Autodesk Inventor part; units mm, degrees
ref_plane "YZ Plane" through (0, 0, 0) normal (1, 0, 0) x (0, 1, 0)
ref_plane "XZ Plane" through (0, 0, 0) normal (0, 1, 0) x (-1, 0, 0)
ref_plane "XY Plane" through (0, 0, 0) normal (0, 0, 1) x (1, 0, 0)
sketch "Sketch1" plane through (0, 0, 0) normal (1, 0, 0) x (0, 1, 0)
  line L0 (2.5746, 9.4872) -> (-17.4254, 9.4872)
  line L1 (-17.4254, 9.4872) -> (-17.4254, -4.5128)
  line L2 (-17.4254, -4.5128) -> (2.5746, -4.5128)
  line L3 (2.5746, -4.5128) -> (2.5746, 9.4872)
  line L4 (2.5746, -4.5128) -> (-9.4254, -4.5128)
  line L5 (-9.4254, -4.5128) -> (-9.4254, -7.5128)
  line L6 (-9.4254, -7.5128) -> (2.5746, -7.5128)
  line L7 (2.5746, -7.5128) -> (2.5746, -4.5128)
  line L8 (2.5746, 9.4872) -> (-9.4254, 9.4872)
  line L9 (-9.4254, 9.4872) -> (-9.4254, 12.4872)
  line L10 (-9.4254, 12.4872) -> (2.5746, 12.4872)
  line L11 (2.5746, 12.4872) -> (2.5746, 9.4872)
  point P0 (0, 0)
  dimension "d0" = 20
  dimension "d1" = 14
  dimension "d2" = 12
  dimension "d3" = 3
  dimension "d4" = 12
  dimension "d5" = 3
extrude "Extrusion1" add sketch "Sketch1" along normal blind 6
sketch "Sketch2" plane through (6, 0, 0) normal (1, 0, 0) x (0, 0, -1)
  circle A0 centre (-2.4872, -11.8754) radius 2.3
  line L0 (-9.4872, -17.4254) -> (4.5128, -17.4254)
  line L1 (-9.4872, -9.4254) -> (-9.4872, -17.4254)
  point P0 (0, 0)
  dimension "d8" = 4.6
  dimension "d9" = 5.55
  dimension "d10" = 7
extrude "Extrusion2" cut sketch "Sketch2" against normal blind 6
sketch "Sketch3" plane through (6, 0, 0) normal (1, 0, 0) x (0, 0, -1)
  line L0 (-5.4872, -17.4254) -> (0.5128, -17.4254)
  line L1 (0.5128, -17.4254) -> (0.5128, -23.4254)
  line L2 (0.5128, -23.4254) -> (-5.4872, -23.4254)
  line L3 (-5.4872, -23.4254) -> (-5.4872, -17.4254)
  line L4 (-9.4872, -9.4254) -> (-9.4872, -17.4254) construction
  line L5 (-9.4872, -17.4254) -> (-5.4872, -17.4254) construction
  line L6 (0.5128, -17.4254) -> (4.5128, -17.4254) construction
  line L7 (-9.4872, -17.4254) -> (4.5128, -17.4254) construction
  point P0 (0, 0)
  dimension "d13" = 6
  dimension "d14" = 6
extrude "Extrusion3" add sketch "Sketch3" against normal blind 6
properties part number "apoio do meioesse"
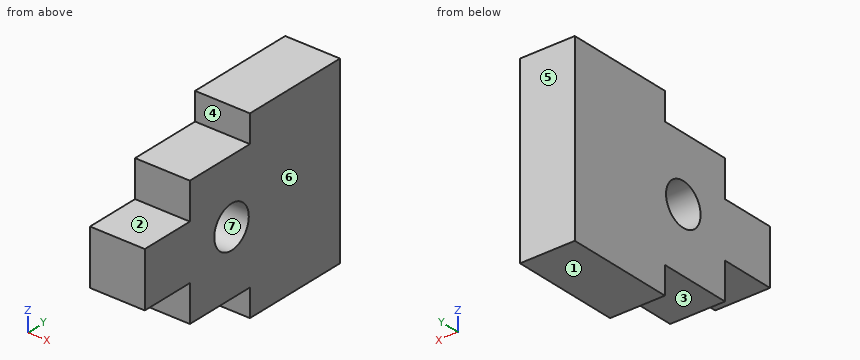
Source: CAD feature listing. Evaluate the final solid. Frame: model axes, mm. Face numbers are marked on the shaded views. A direction names the side the tool comes from. Give positions to 0.01 mm unless a question says otherwise; leave off trailing zeros. Write each loop counter-clockwise with the first axis right and the second up, starting at its lowest first coordinate (ties: lowest second). Pieces come first, ordered by that corner, then holes. Notation, with made-up numbers: M 44.25,-3.75 L 52.25,-3.75 A23 ccw 52.25,26.25 Z; hole C -34.75,58.25 d1. An arc over 180 degrees is marked long. Return JSON: item names as keys, results as strings. Group by question number.
1) Cut plane A-A, the plane x = 1.1. Output: boundary loops of the cut face in (y, z).
2) Cut plane B-B, the plane z = 0.75. Output: boundary loops of the cut face in (x, y).
3) Ray query, L1, parallel to Y at x = 5, z = -0.75; L2, parallel to Z at x = 5.55, y = -22.5; L3, parallel to Y at x = 3.25, z = 11. Return the intervals inside material, ascending.
4) First-contact query: pin 1 Ø2.5 at (x, z) = (4.5, 10.5) entering from -Y; pin 2 Ø3 at (x, y) = (3.5, -12.5) entering from -Z; pin 3 Ø1.5 at (x, y) = (4, -13) entering from +Z. Flat tips, straight axial feed; report the tip coordinate or a pass-through.
5) Cut plane C-C, the plane y = -12.5. Output: boundary loops of the cut face in (x, z), then the cut area to 3 significant figures.
6) Set-up query: the marked faces 1, 2 and 3. Return all of +Z, -Z, +X, -X, +Y, -Y with unobstructed straight access to the full face (end or side cutting, diameter ignored); none if empty.
7) Draft query along Y for the marked faces 4, 5, 6 and 7. Return one class per face: released by +Y, released by -Y, zero draft, split by the parting line, or undercut.
8) Cut plane D-D, the plane z = 8.5. Output: boundary loops of the cut face in (x, y), then the cut area to 3 significant figures.
Data:
{
 "1": {"outline": "M -23.43,-0.51 L -17.43,-0.51 L -17.43,-4.51 L -9.43,-4.51 L -9.43,-7.51 L 2.57,-7.51 L 2.57,12.49 L -9.43,12.49 L -9.43,9.49 L -17.43,9.49 L -17.43,5.49 L -23.43,5.49 Z; hole C -11.88,2.49 d4.6"},
 "2": {"outline": "M 0,-23.43 L 6,-23.43 L 6,-13.38 L 0,-13.38 Z; M 0,-10.37 L 6,-10.37 L 6,2.57 L 0,2.57 Z"},
 "3": {"L1": "y = -17.43 to 2.57", "L2": "z = -0.51 to 5.49", "L3": "y = -9.43 to 2.57"},
 "4": {"pin 1": "stops at y = -17.43", "pin 2": "stops at z = -4.51", "pin 3": "stops at z = 9.49"},
 "5": {"outline": "M 0,-4.51 L 6,-4.51 L 6,0.27 L 0,0.27 Z; M 0,4.7 L 6,4.7 L 6,9.49 L 0,9.49 Z", "area": "57.4 mm²"},
 "6": {"face 1": "-Z, +X, -X, +Y, -Y", "face 2": "+Z, +X, -X, -Y", "face 3": "-Z, +X, -X, -Y"},
 "7": {"face 4": "released by -Y", "face 5": "released by +Y", "face 6": "zero draft", "face 7": "undercut"},
 "8": {"outline": "M 0,-17.43 L 6,-17.43 L 6,2.57 L 0,2.57 Z", "area": "120 mm²"}
}
